Input: part model. Units: mm. Frame: model coordinates. Face numbers are marked on the shaded views. Coordinates: 2 decimals unless noted, no trailing zeros. Loops run counter-clockwise (first coordinate to the right, second up) from the corner with the lowest first, then second, coordinate; pieces in that order, holes last.
(1) Contact query for a flat-ended pin moving along its axis: P1, Ø1.5, axis at y = 18, z = -7, coming from the +X side. Output: stop coordinate, or through.
(2) Mould query, pull axis Z, two halves, no side actions, for the marked faces 1, 2 and 3. Classes: released by +Z, released by -Z, zero draft, split by the parting line, or undercut.
(3) Section A-A, the plane x = 0. Return loops of the section in (y, z), then the cut area to 3 significant figures.
(4) Section B-B, the plane y = 18.35. Return loops of the section in (x, z), then the cut area to 3 significant figures.
(5) Section C-C, the plane z = 7. Return loops of the section in (x, y), then the cut area to 3 significant figures.
(6) Line query: L1, parallel to Z at x = -0.25, y = 19.05; L2, parallel to X at y = 19.05, z = -3.25; L3, parallel to Z at x = 7.5, y = 17.7. Output: solid intervals per line, ascending.
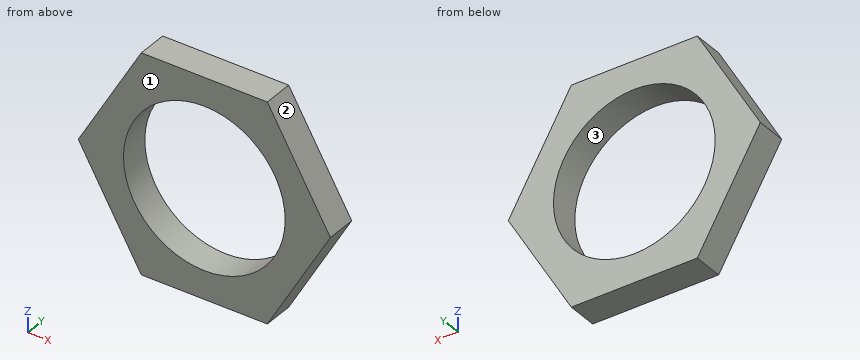
```python
from build123d import *

# Parameters (mm, degrees)
NUT_DEPTH     = 3.2
BORE_SKETCH_W = 8.52
BORE_SKETCH_H = 5.2


with BuildPart() as part:
    # Nut Sketch → Nut (new body)
    with BuildSketch(Plane(origin=(0, 17.2, 0), x_dir=(1, 0, 0), z_dir=(0, 1, 0))):
        Polygon((13.279056191, 0), (6.639528096, 11.5), (-6.639528096, 11.5), (-13.279056191, 0), (-6.639528096, -11.5), (6.639528096, -11.5), align=None)
    extrude(amount=NUT_DEPTH)

    # Bore Sketch → Bore (revolve, cut)
    with BuildSketch(Plane.XY, mode=Mode.PRIVATE) as bore_sk:
        with Locations((4.26, 18.8)):
            Rectangle(BORE_SKETCH_W, BORE_SKETCH_H)
    revolve(bore_sk.sketch.rotate(Axis((0, -100, 0), (0, 1, 0)), 270), axis=Axis((0, -100, 0), (0, 1, 0)), mode=Mode.SUBTRACT)


solid = part.part
```
Report:
1. P1: stops at x = 9.67
2. face 1: zero draft
2. face 2: released by +Z
2. face 3: undercut
3. outline: (17.2, -11.5) - (20.4, -11.5) - (20.4, -8.52) - (17.2, -8.52) - close; (17.2, 8.52) - (20.4, 8.52) - (20.4, 11.5) - (17.2, 11.5) - close
3. area: 19.1 mm2
4. outline: (-13.28, 0) - (-6.64, -11.5) - (6.64, -11.5) - (13.28, 0) - (6.64, 11.5) - (-6.64, 11.5) - close; hole circle Ø17.04 at (0, 0)
4. area: 230 mm2
5. outline: (-9.24, 17.2) - (-4.86, 17.2) - (-4.86, 20.4) - (-9.24, 20.4) - close; (4.86, 17.2) - (9.24, 17.2) - (9.24, 20.4) - (4.86, 20.4) - close
5. area: 28.0 mm2
6. L1: z = -11.5 to -8.52, 8.52 to 11.5
6. L2: x = -11.4 to -7.88, 7.88 to 11.4
6. L3: z = -10.01 to -4.04, 4.04 to 10.01
